Autodesk Inventor part; units mm, degrees
ref_plane "YZ Plane" through (0, 0, 0) normal (1, 0, 0) x (0, 1, 0)
ref_plane "XZ Plane" through (0, 0, 0) normal (0, 1, 0) x (-1, 0, 0)
ref_plane "XY Plane" through (0, 0, 0) normal (0, 0, 1) x (1, 0, 0)
sketch "Sketch1" plane through (0, 0, 0) normal (0, 0, 1) x (1, 0, 0)
  circle A0 centre (0, 0) radius 12
  dimension "d0" = 24
extrude "Extrusion1" add sketch "Sketch1" along normal blind 68.5
sketch "Sketch2" plane through (0, 0, 68.5) normal (0, 0, 1) x (1, 0, 0)
  circle A0 centre (0, 0) radius 3.5
  dimension "d3" = 7
extrude "Extrusion2" add sketch "Sketch2" along normal blind 2.25
sketch "Sketch3" plane through (0, 0, 70.75) normal (0, 0, 1) x (1, 0, 0)
  circle A0 centre (0, 0) radius 3.5
  circle A1 centre (0, 0) radius 2
  dimension "d6" = 4
extrude "Extrusion3" add sketch "Sketch3" along normal blind 10 contours A1
properties part number "Motor_elevation"
Can you work these out from the model? Positions are in its coordinate system, mm. A direction names the side the tool comes from. Give positions to 0.01 mm unless a question says otherwise; leave off trailing zeros. Loops run counter-clockwise (first coordinate to the right, second up) from the corner with the lowest first, then second, coordinate; pieces in that order, holes last. Notation, with made-up numbers: (80.25, -30.5) -> (103.25, -30.5) arc R23 ccw to (103.25, -0.5) -> close; hole circle Ø6 at (-20.75, 72). An arc over 180 degrees is marked (long way). Use one line per item in the form item = value.
1) If we section it at D-D (y = 4.25): Please give me the cut outline in (x, z), plus the area to 3 significant figures.
Answers:
outline = (-11.22, 0) -> (11.22, 0) -> (11.22, 68.5) -> (-11.22, 68.5) -> close
area = 1,540 mm²
2) If we section it at C-C (z = 22): Please give me the cut outline in (x, y).
Answers:
outline = circle Ø24 at (0, 0)
3) For faces 1 (the face through (0, 0, 0)), 2 (the face through (3.233, 1.341, 69.609)), which set-ups out of +Z, -Z, +X, -X, +Y, -Y let a thin tool reach every point of the face, with its end or its side?
Answers:
face_1 = -Z, +X, -X, +Y, -Y
face_2 = +Z
4) If we section it at A-A (y = 0): Please give me the cut outline in (x, z).
Answers:
outline = (-12, 0) -> (12, 0) -> (12, 68.5) -> (3.5, 68.5) -> (3.5, 70.75) -> (2, 70.75) -> (2, 80.75) -> (-2, 80.75) -> (-2, 70.75) -> (-3.5, 70.75) -> (-3.5, 68.5) -> (-12, 68.5) -> close
5) Will these pins go through, and if not, where does the flat tip stop? pin 1 (2 mm diameter, centred on y = -4, z = 59.5, fed in from -X); pin 2 (1 mm diameter, centred on y = -5, z = 60.5, fed in from +X); pin 3 (2 mm diameter, centred on x = -7, y = -8.5, fed in from +Z).
Answers:
pin_1 = -11.62
pin_2 = 11.12
pin_3 = 68.5
6) I need wall thicknesses on line 1 along Z through (x, y) = (4.25, -10.5); line 2 along X through (y, z) = (-0.25, 7.5); line 3 along Y through (x, z) = (2, 32.5). Which ranges of each line are inside material? Lowest first, please.
Answers:
line_1 = 0 to 68.5
line_2 = -12 to 12
line_3 = -11.83 to 11.83
